```python
from build123d import *

# Parameters (mm, degrees)
SKETCH1_R           = 50.8
BOSS_EXTRUDE1_DEPTH = 25
FILLET2_R           = 8
FILLET3_R           = 8
SKETCH2_R           = 15
BOSS_EXTRUDE2_DEPTH = 5
SKETCH3_R           = 12
CUT_EXTRUDE1_DEPTH  = 25
FILLET4_R           = 8
SKETCH5_R           = 1.61
SKETCH5_R_2         = 4.2
CUT_EXTRUDE2_DEPTH  = 78.85422275
CUT_EXTRUDE3_DEPTH  = 78.85422275
SKETCH7_R           = 3.4
CUT_EXTRUDE4_DEPTH  = 2.3


with BuildPart() as part:
    # Sketch1 → Boss-Extrude1 (new body)
    with BuildSketch(Plane(origin=(0, 0, 0), x_dir=(1, 0, 0), z_dir=(0, 1, 0))):
        with Locations(Location((0, 0, 0), (0, 0, 270))):
            Circle(SKETCH1_R)
    extrude(amount=BOSS_EXTRUDE1_DEPTH)

    # Fillet2
    fillet2_edges = [part.edges().sort_by_distance(p)[0] for p in [
        (0, 25, -50.8),
    ]]
    fillet(fillet2_edges, radius=FILLET2_R)

    # Fillet3
    fillet3_edges = [part.edges().sort_by_distance(p)[0] for p in [
        (0, 0, -50.8),
    ]]
    fillet(fillet3_edges, radius=FILLET3_R)

    # Sketch2 → Boss-Extrude2 (add)
    with BuildSketch(Plane.XZ):
        with Locations(Location((0, 0, 0), (0, 0, 90))):
            Circle(SKETCH2_R)
    extrude(amount=BOSS_EXTRUDE2_DEPTH)

    # Sketch3 → Cut-Extrude1 (cut)
    with BuildSketch(Plane(origin=(0, 25, 0), x_dir=(1, 0, 0), z_dir=(0, 1, 0))):
        with Locations(Location((0, 0, 0), (0, 0, 270))):
            Circle(SKETCH3_R)
    extrude(amount=-CUT_EXTRUDE1_DEPTH, mode=Mode.SUBTRACT)

    # Fillet4
    # the kernel refuses this fillet: 8 mm, written as the material it adds along each edge
    with BuildSketch(Plane(origin=(0, 0, 0), x_dir=(0, 0, 1), z_dir=(1, 0, 0))) as fillet4_piece_1:
        with BuildLine():
            CenterArc((22.416198487, 8), FILLET4_R, 202.024312837, 67.975687163)
            Line((15, 5), (14.85167603, 4.94))
            ThreePointArc((14.85167603, 4.94), (14.84, 2.5), (14.84, 0))
            Line((14.84, 0), (15, -0.16))
            Line((15, -0.16), (22.416198487, -0.16))
            Line((22.416198487, -0.16), (22.416198487, 0))
        make_face()
    revolve(axis=Axis((0, 0, 0), (0, -1, 0)))

    # Sketch5 → Cut-Extrude2 (cut, through all)
    with BuildSketch(Plane.XZ.offset(5)):
        with Locations(Location((0, 8, 0), (0, 0, 270))):
            Circle(SKETCH5_R)
        with Locations(Location((0, -8, 0), (0, 0, 90))):
            Circle(SKETCH5_R)
        with Locations(Location((8, 0, 0), (0, 0, 270))):
            Circle(SKETCH5_R)
        with Locations(Location((-8, 0, 0), (0, 0, 90))):
            Circle(SKETCH5_R)
        with Locations(Location((0, 0, 0), (0, 0, 270))):
            Circle(SKETCH5_R_2)
    extrude(amount=-CUT_EXTRUDE2_DEPTH, mode=Mode.SUBTRACT)

    # Sketch6 → Cut-Extrude3 (cut, through all)
    with BuildSketch(Plane(origin=(0, 25, 0), x_dir=(1, 0, 0), z_dir=(0, 1, 0))):
        with BuildLine():
            Line((6.669640143, 14.619160774), (17.119775233, 37.524775128))
            ThreePointArc((17.119775233, 37.524775128), (-2.42176691, 41.174391282), (-21.4007271, 35.259102825))
            Line((-21.4007271, 35.259102825), (-8.337442905, 13.736484528))
            ThreePointArc((-8.337442905, 13.736484528), (-0.943488661, 16.041003414), (6.669640143, 14.619160774))
        make_face()
        with BuildLine():
            Line((13.736484528, 8.337442905), (35.259102825, 21.4007271))
            ThreePointArc((35.259102825, 21.4007271), (41.174391282, 2.42176691), (37.524775128, -17.119775233))
            Line((37.524775128, -17.119775233), (14.619160774, -6.669640143))
            ThreePointArc((14.619160774, -6.669640143), (16.041003414, 0.943488661), (13.736484528, 8.337442905))
        make_face()
        with BuildLine():
            Line((8.337442905, -13.736484528), (21.4007271, -35.259102825))
            ThreePointArc((21.4007271, -35.259102825), (2.42176691, -41.174391282), (-17.119775233, -37.524775128))
            Line((-17.119775233, -37.524775128), (-6.669640143, -14.619160774))
            ThreePointArc((-6.669640143, -14.619160774), (0.943488661, -16.041003414), (8.337442905, -13.736484528))
        make_face()
        with BuildLine():
            Line((-13.736484528, -8.337442905), (-35.259102825, -21.4007271))
            ThreePointArc((-35.259102825, -21.4007271), (-41.174391282, -2.42176691), (-37.524775128, 17.119775233))
            Line((-37.524775128, 17.119775233), (-14.619160774, 6.669640143))
            ThreePointArc((-14.619160774, 6.669640143), (-16.041003414, -0.943488661), (-13.736484528, -8.337442905))
        make_face()
    extrude(amount=-CUT_EXTRUDE3_DEPTH, mode=Mode.SUBTRACT)

    # Sketch7 → Cut-Extrude4 (cut)
    with BuildSketch(Plane(origin=(0, 0, 0), x_dir=(1, 0, 0), z_dir=(0, 1, 0))):
        with Locations(Location((-8, 0, 0), (0, 0, 270))):
            Circle(SKETCH7_R)
        with Locations(Location((0, 8, 0), (0, 0, 270))):
            Circle(SKETCH7_R)
        with Locations(Location((8, 0, 0), (0, 0, 270))):
            Circle(SKETCH7_R)
        with Locations(Location((0, -8, 0), (0, 0, 270))):
            Circle(SKETCH7_R)
    extrude(amount=-CUT_EXTRUDE4_DEPTH, mode=Mode.SUBTRACT)


solid = part.part
```
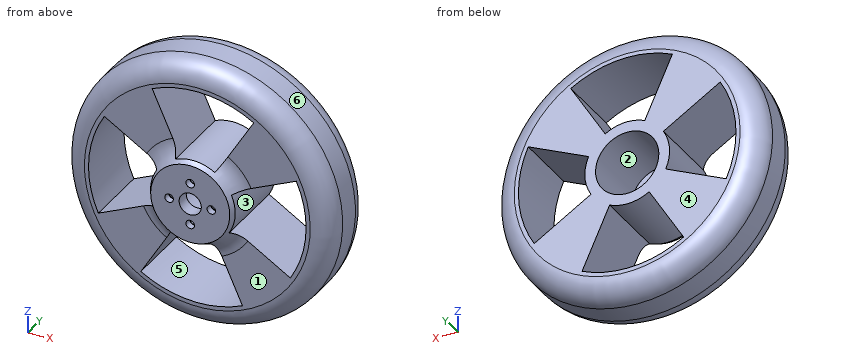
The listing builds one solid part. Answer for the finished solid, in the listing's coordinates (mm). Face numbers are marked on the shaded views. A direction names the side the tool comes from. Give positions to 0.01 mm unless a question says otherwise; leave off trailing zeros. Order: outer loops, then holes, each group sorted by start corner. A loop starts at its lowest first (then second) coordinate and runs counter-clockwise, first axis right, second up. Notation, with made-up numbers: (68, 84) -> (111, 84) arc R20 cw to (111, 90) -> close; hole circle Ø8 at (32, -4). An arc over 180 degrees is marked (long way). Answer as a JSON object with one key per item and string values. Group by question number.
Item 1: Determine the mould class of the marked faces 4, 5 and 6 for opening direction Z: pulls with the +Z half, pulls with the -Z half, needs draft (parallel to the pull), parting line crosses it, or undercut.
Item 2: Consider L1, parallel to X at y = -3, z = 0; L2, parallel to X at y = 23.5, z = 0.5; L3, parallel to Z at x = -19.5, y = 21. Determine where each line is inside the solid, lowest interval first. Write a range as from..to.
Item 3: The part is cut by section B-B on y = 2. Write down the section's boundary in (x, z), and give its area (3 significant figures).
Item 4: A tool of negligible diameter and unlimited length cuts with its end or side. For the marked faces 1, 2 and 3, from which of +Z, -Z, +X, -X, +Y, -Y can it reach the whole face along a straight path? Write none if from no direction.
Item 5: The part is cut by section A-A on z = 0. Give the number of separate pieces and of enclosed holes in the cut face, and give its area (3 significant figures).
Item 6: Flat-ended cylindrical pins translate along their axes: pin 1 (5.5 mm diameter, centred on x = 8.5, z = 1.5, fed in from +Y); pin 2 (1.5 mm diameter, centred on y = 14, z = 37.5, fed in from -X); pin 3 (6 mm diameter, centred on y = 3.5, z = 29.5, fed in from +X). Find the tip coordinate at first contact, or state that the pin passes through.
Result set:
{
 "1": {"face 4": "needs draft", "face 5": "undercut", "face 6": "parting line crosses it"},
 "2": {"L1": "-16.07..-9.61, -6.39..-4.2, 4.2..6.39, 9.61..16.07", "L2": "-47.46..-41.24, -16.06..-11.99, 11.99..16.06, 41.24..47.46", "L3": "-45.75..-36.34, -32.13..-8.9, 11.84..45.75"},
 "3": {"outline": "circle Ø96.18 at (0, 0); hole (-37.52, -17.12) -> (-14.62, -6.67) arc R16.07 cw to (-13.74, 8.34) -> (-35.26, 21.4) arc R41.25 ccw to start; hole (-21.4, -35.26) arc R41.25 ccw to (17.12, -37.52) -> (6.67, -14.62) arc R16.07 cw to (-8.34, -13.74) -> close; hole (-17.12, 37.52) -> (-6.67, 14.62) arc R16.07 cw to (8.34, 13.74) -> (21.4, 35.26) arc R41.25 ccw to start; hole circle Ø24 at (0, 0); hole (13.74, -8.34) -> (35.26, -21.4) arc R41.25 ccw to (37.52, 17.12) -> (14.62, 6.67) arc R16.07 cw to start", "area": "4,000 mm²"},
 "4": {"face 1": "-Y", "face 2": "+Y", "face 3": "+Y, -Y"},
 "5": {"separate pieces": "6", "enclosed holes": "0", "area": "694 mm²"},
 "6": {"pin 1": "y = 0", "pin 2": "x = -35.07", "pin 3": "x = 42.41"}
}
